Verification items for the finished model (mm, model axes). Face numbers are marked on the shaded views. A direction names the side the tool comes from. Give positions to 0.01 mm unless a question says otherwise; leave off trailing zeros. Write each loop counter-clockwise with the first axis right and the second up, starting at its lowest first coordinate (ties: lowest second). Pieces come first, ordered by that corner, then holes. Notation, with made-up numbers: (67, 27.25) -> (80, 27.25) arc R21 ccw to (80, 65.25) -> close; hole circle Ø8 at (53.25, 51.5). An arc over 180 degrees is marked (long way). Answer as CSV lines item,"result".
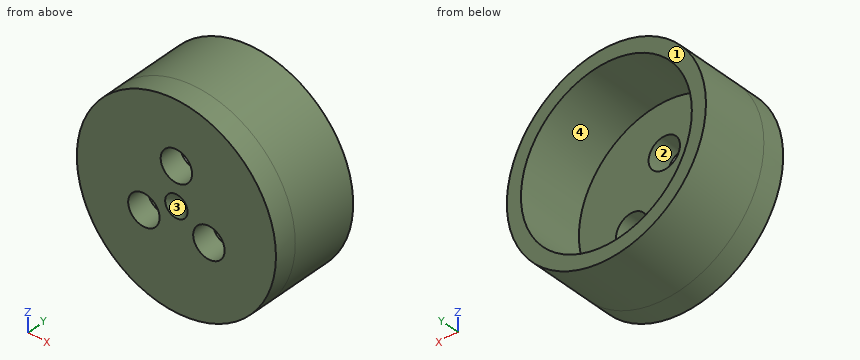
```python
from build123d import *

# Parameters (mm, degrees)
F0_R           = 44.4
F1_DEPTH       = 10
F2_R           = 44.4
F2_R_2         = 38.1
F3_DEPTH       = 30
F4_R           = 7
F5_DEPTH       = 40.001
F7_D           = 0.02
F7_DEPTH       = 5
F7_CSINK_D     = 10
F7_CSINK_ANGLE = 90
F7_TIP         = 0.0060086062


with BuildPart() as f1:
    # F0 (on Front) → F1 (new body)
    with BuildSketch(Plane.XZ):
        Circle(F0_R)
    extrude(amount=F1_DEPTH)

    # F2 (on face) → F3 (join)
    with BuildSketch(Plane(origin=(0, 0, 0), x_dir=(-1, 0, 0), z_dir=(0, 1, 0))):
        Circle(F2_R)
        Circle(F2_R_2, mode=Mode.SUBTRACT)
    extrude(amount=F3_DEPTH)

    # F4 (on face) → F5 (cut, through all)
    with BuildSketch(Plane.XZ.offset(10)):
        with Locations((0, 16.7431578065)):
            Circle(F4_R)
        with Locations((-14.5, -8.3715789032)):
            Circle(F4_R)
        with Locations((14.5, -8.3715789032)):
            Circle(F4_R)
    extrude(amount=-F5_DEPTH, mode=Mode.SUBTRACT)

    # F7
    with Locations(Plane.XZ.offset(10)):
        with Locations((0, 0)):
            CounterSinkHole(F7_D / 2, F7_CSINK_D / 2, depth=F7_DEPTH, counter_sink_angle=F7_CSINK_ANGLE)
            with Locations((0, 0, -(F7_DEPTH + F7_TIP / 2))):  # 118° drill point
                Cone(0, F7_D / 2, F7_TIP, mode=Mode.SUBTRACT)


solid = f1.part
```
1) Draft check along X on the marked faces 1 and 2. Enter one of: +X half, -X half, draft (parallel to the pull), parting line (faces both ways), or undercut.
Reported:
face 1,"draft"
face 2,"undercut"
2) Scan lines: line 1 along Z through (x, y) = (0, 23); line 2 along Y through (x, z) = (25, -24); line 3 along Z through (x, y) = (0, -4.95). Record each from-to range of solid material in increasing order.
Reported:
line 1,"-44.4 to -38.1, 38.1 to 44.4"
line 2,"-10 to 0"
line 3,"-44.4 to 9.74, 23.74 to 44.4"
3) Section check A-A (z = 19). Record the boundary of the cut face in (x, y).
Reported:
outline,"(-40.13, -10) -> (-6.63, -10) -> (-6.63, 0) -> (-33.02, 0) -> (-33.02, 30) -> (-40.13, 30) -> close; (6.63, -10) -> (40.13, -10) -> (40.13, 30) -> (33.02, 30) -> (33.02, 0) -> (6.63, 0) -> close"
4) Depth check by flat-ended pin: pin 1 (3 mm diameter, centred on y = -1.5, z = 32.5, fed in from +X); pin 2 (1.5 mm diameter, centred on y = 14, z = -25.5, fed in from -X); pin 3 (18 mm diameter, centred on x = 0, z = 16.74, fed in from +Y). Enter the tip coordinate at first touch or a pass-through.
Reported:
pin 1,"x = 31.79"
pin 2,"x = -36.86"
pin 3,"y = 0"
5) Tool access check on the marked faces 3 and 4. Record the directions out of +Z, -Z, +X, -X, +Y, -Y that give a thin tool (end or side, any length) a straight path to the whole face; none if there is none.
Reported:
face 3,"-Y"
face 4,"+Y"
6) Section check D-D (x = 33.5). Record the boundary of the cut face in (y, z).
Reported:
outline,"(-10, -29.14) -> (30, -29.14) -> (30, -18.15) -> (0, -18.15) -> (0, 18.15) -> (30, 18.15) -> (30, 29.14) -> (-10, 29.14) -> close"
7) Section check B-B (x = -14.5). Record the boundary of the cut face in (y, z).
Reported:
outline,"(-10, -41.97) -> (30, -41.97) -> (30, -35.23) -> (0, -35.23) -> (0, -15.37) -> (-10, -15.37) -> close; (-10, -1.37) -> (0, -1.37) -> (0, 35.23) -> (30, 35.23) -> (30, 41.97) -> (-10, 41.97) -> close"
8) Section check C-C (y = 17.5). Record the boundary of the cut face in (x, z).
Reported:
outline,"circle Ø88.8 at (0, 0); hole circle Ø76.2 at (0, 0)"
